Input: part model. Units: mm. Frame: model coordinates. A direction names the side the tool comes from. Give positions to 0.01 mm unless a question says otherwise; leave off trailing zeros. Order: outer loops, then holes, each group sorted by start corner. A loop starts at its lowest first (then second) coordinate and runs counter-clockwise, first axis right, second up. Notation, with made-up numbers: (-13, -18) - (9, -18) arc R20 cw to (9, 7) - close; hole circle Ø3 at (18.5, 15). An arc over 180 degrees is marked (long way). Answer in a Markdown table with one row per item. Add a question column.
1. Section query B-B on y = 0. Return loops of the section in (x, z), and give its area (3 significant figures).
2. Section query A-A on z = 17. Return loops of the section in (x, y).
3. Ray query, line 1 (X direction, y = 0.1, z = 12); line 2 (Z direction, x = 1.4, y = 0.65); line 3 (Y direction, x = -0.15, z = 28). Return the intervals inside material, ascending. Write a range as [from, to].
4. Contact query for flat-ended pins moving along their axis: pin 1 (2 mm diameter, centred on y = 2, z = 25.5, fed in from -X); pin 2 (0.8 mm diameter, centred on x = -0.5, y = 0.5, fed in from -Z). Output: stop coordinate, or through.
5. Access query for faces 1 (the face through (0, -2, 0)), 2 (the face through (0, 0, -1.7)), 3 (the face through (0, 0, 35)). Directions: +Z, -Z, +X, -X, +Y, -Y. A direction counts if a zero-diameter tool reaches every point of the face in a straight line with its end or side. Return the directions, or none.
6. Mould query, pull axis Y, two halves, no side actions, for faces 4 (the face through (1.1, -1.1, -3)), 5 (the face through (-0.596, -2.685, -1.482)), 6 (the face through (-0.619, 1.086, -2.359)). Classes: released by +Y, released by -Y, zero draft, split by the parting line, or undercut.
```python
from build123d import *

# Parameters (mm, degrees)
F0_R     = 1.5
F1_DEPTH = 35
F2_R     = 2.75
F3_DEPTH = 3
F5_DEPTH = 1.3
F6_SIZE  = 0.25


with BuildPart() as f1:
    # F0 (on Top) → F1 (new body)
    with BuildSketch(Plane.XY):
        Circle(F0_R)
    extrude(amount=F1_DEPTH)

    # F2 (on Top) → F3 (join)
    with BuildSketch(Plane.XY):
        Circle(F2_R)
    extrude(amount=-F3_DEPTH)

    # F4 (on face) → F5 (cut)
    with BuildSketch(Plane(origin=(0, 0, -3), x_dir=(1, 0, 0), z_dir=(0, 0, -1))):
        Polygon((0.019386, -1.443245), (1.25958, -0.704834), (1.240194, 0.738412), (-0.019386, 1.443245), (-1.25958, 0.704834), (-1.240194, -0.738412), align=None)
    extrude(amount=-F5_DEPTH, mode=Mode.SUBTRACT)

    # F6
    f6_edges = [f1.edges().sort_by_distance(p)[0] for p in [
        (-2.75, 0, -3),
        (-2.75, 0, 0),
        (-1.5, 0, 35),
    ]]
    chamfer(f6_edges, length=F6_SIZE)


solid = f1.part
```
Answer:
| question | item | result |
|---|---|---|
| 1 | outline | (-2.75, -2.75) - (-2.5, -3) - (-1.25, -3) - (-1.25, -1.7) - (1.25, -1.7) - (1.25, -3) - (2.5, -3) - (2.75, -2.75) - (2.75, -0.25) - (2.5, 0) - (1.5, 0) - (1.5, 34.75) - (1.25, 35) - (-1.25, 35) - (-1.5, 34.75) - (-1.5, 0) - (-2.5, 0) - (-2.75, -0.25) - close |
| 1 | area | 118 mm² |
| 2 | outline | circle Ø3 at (0, 0) |
| 3 | line 1 | x = [-1.5, 1.5] |
| 3 | line 2 | z = [-3, 0] |
| 3 | line 3 | y = [-1.49, 1.49] |
| 4 | pin 1 | stops at x = -1.12 |
| 4 | pin 2 | stops at z = -1.7 |
| 5 | face 1 | +Z |
| 5 | face 2 | -Z |
| 5 | face 3 | +Z, +X, -X, +Y, -Y |
| 6 | face 4 | zero draft |
| 6 | face 5 | split by the parting line |
| 6 | face 6 | undercut |
